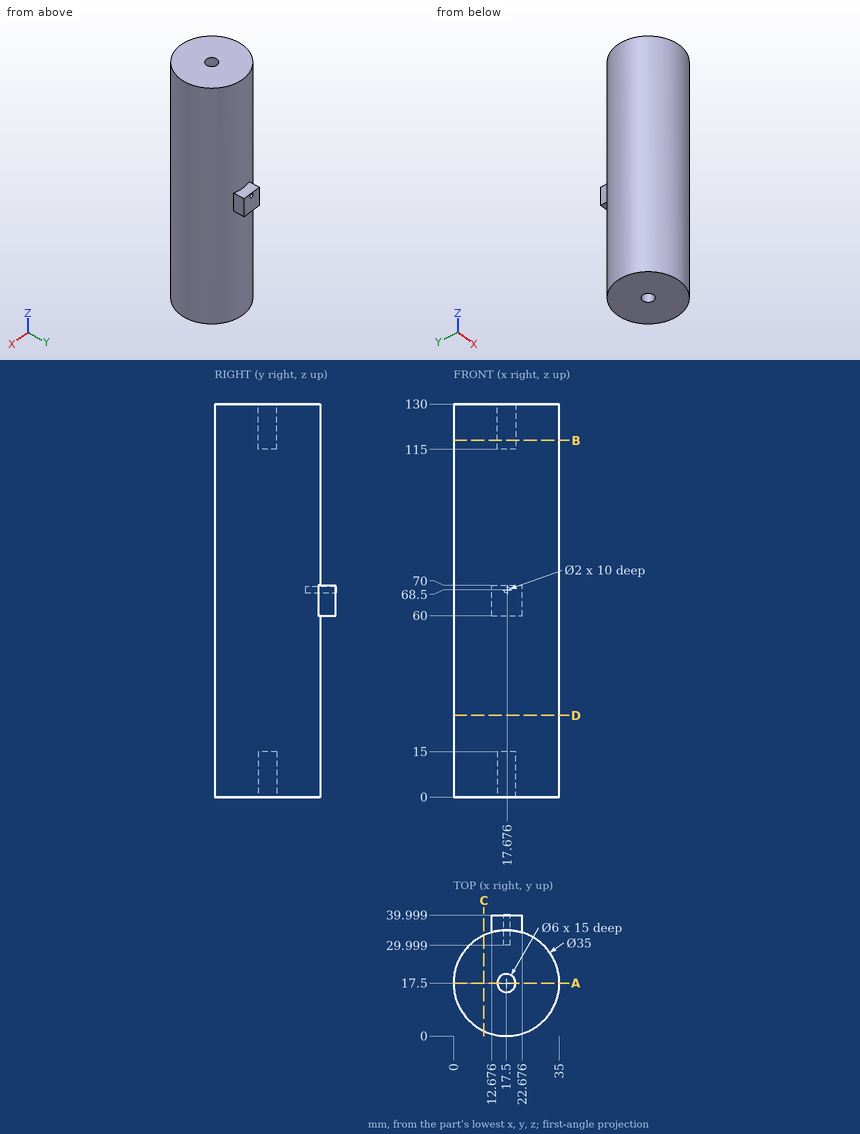
Could you check a few things on this drawing? It's one solid part, dimensions in mm from its lowest x, y, z. Give positions to 0.01 mm unless a question says otherwise; leave off trailing zeros. Write each loop counter-clockwise with the first axis right and the second up, starting at its lowest first coordinate (ties: lowest second). Pieces come first, ordered by that corner, then holes. Notation, with made-up numbers: M 61,-33 L 117,-33 A26 cw 117,-18 Z; hole C 66,4.25 d9. An arc over 180 degrees is marked long. Put each result on its own line as item: value. Start each with the question number.
Item 1: Will these pins go through, and if not, where does the flat tip stop? pin 1 (4.5 mm diameter, centred on y = 37, z = 63, fed in from +X); pin 2 (1.5 mm diameter, centred on x = 18, z = 39, fed in from +Y); pin 3 (3.5 mm diameter, centred on x = 17.5, y = 17.5, fed in from +Z).
Item 2: I need wall thicknesses on L1, parallel to Y at x = 17.5, z = 11.75; L2, parallel to X at y = 17, z = 119; L3, parallel to Y at x = 16.5, z = 36.5. Which ranges of each line are inside material? Lowest first, please. Write a range as from..to.
Item 3: If we section it at A-A, the plane y = 17.5: Write out the boundary of the cut face in (x, z), then the cut area to 3 significant figures.
Item 4: If we section it at D-D, the plane z = 27: Write out the boundary of the cut face in (x, y), then the cut area to 3 significant figures.
Item 5: If we section it at B-B, the plane z = 118: Write out the boundary of the cut face in (x, y), then the cut area to 3 significant figures.
Item 6: If we section it at C-C, the plane x = 10: Write out the boundary of the cut face in (y, z).
Values:
1. pin 1: x = 22.68
1. pin 2: y = 35
1. pin 3: z = 115
2. L1: 0..14.5, 20.5..35
2. L2: 0.01..14.54, 20.46..34.99
2. L3: 0.03..34.97
3. outline: M 0,0 L 14.5,0 L 14.5,15 L 20.5,15 L 20.5,0 L 35,0 L 35,130 L 20.5,130 L 20.5,115 L 14.5,115 L 14.5,130 L 0,130 Z
3. area: 4,370 mm²
4. outline: C 17.5,17.5 d35
4. area: 962 mm²
5. outline: C 17.5,17.5 d35; hole C 17.5,17.5 d6
5. area: 934 mm²
6. outline: M 1.69,0 L 33.31,0 L 33.31,130 L 1.69,130 Z
